Source: CAD feature listing. Evaluate the final solid. Frame: model axes, mm. A direction names the side the tool comes from. Coordinates: 2 decimals unless noted, no trailing zeros. Loops run counter-clockwise (first coordinate to the right, second up) from the corner with the lowest first, then second, coordinate; pieces in that order, holes last.
from build123d import *

# Parameters (mm, degrees)
SKETCH1_R               = 1.6
BOSS_EXTRUDE1_DEPTH     = 17
SKETCH2_R               = 1.65
CUT_EXTRUDE1_DEPTH      = 18
BOSS_EXTRUDE2_OUTLINE_R = 1.6
BOSS_EXTRUDE2_OUTLINE_W = 18.2
BOSS_EXTRUDE2_OUTLINE_H = 15.5
BOSS_EXTRUDE2_DEPTH     = 5
SKETCH5_R               = 8.1
CUT_EXTRUDE2_DEPTH      = 3
SKETCH6_R               = 4.5
CUT_EXTRUDE3_DEPTH      = 96.845918014
BOSS_EXTRUDE4_DEPTH     = 14
BOSS_EXTRUDE5_DEPTH     = 3
FILLET1_R               = 2
SKETCH10_W              = 9
SKETCH10_H              = 15
CUT_EXTRUDE4_DEPTH      = 5
FILLET2_R               = 1
FILLET3_R               = 1
FILLET4_R               = 2


# Read off the part's stored shape, not the designer's step: Boss-Extrude2
with BuildPart() as part:
    # Sketch1 → Boss-Extrude1 (new body)
    with BuildSketch(Plane.XY):
        with BuildLine():
            Line((10, -87.5), (10, -90))
            Line((10, -90), (26.2, -90))
            Line((26.2, -90), (26.2, 0))
            ThreePointArc((26.2, 0), (0, 26.2), (-26.2, 0))
            Line((-26.2, 0), (-26.2, -90))
            Line((-26.2, -90), (-10, -90))
            Line((-10, -90), (-10, -87.5))
            Line((-10, -87.5), (10, -87.5))
        make_face()
        with Locations((-23.7, -87.5)):
            Circle(SKETCH1_R, mode=Mode.SUBTRACT)
        with Locations((23.7, -87.5)):
            Circle(SKETCH1_R, mode=Mode.SUBTRACT)
        with Locations((-23.7, 0)):
            Circle(SKETCH1_R, mode=Mode.SUBTRACT)
        with Locations((0, 23.7)):
            Circle(SKETCH1_R, mode=Mode.SUBTRACT)
        with Locations((23.7, 0)):
            Circle(SKETCH1_R, mode=Mode.SUBTRACT)
        with BuildLine():
            Line((-21.2, -85), (21.2, -85))
            Line((21.2, -85), (21.2, 0))
            ThreePointArc((21.2, 0), (0, 21.2), (-21.2, 0))
            Line((-21.2, 0), (-21.2, -85))
        make_face(mode=Mode.SUBTRACT)
    extrude(amount=BOSS_EXTRUDE1_DEPTH)

    # Sketch2 → Cut-Extrude1 (cut)
    with BuildSketch(Plane.XZ.offset(90)):
        with Locations((15.5, 11.5)):
            Circle(SKETCH2_R)
        with Locations((-15.5, 11.5)):
            Circle(SKETCH2_R)
    extrude(amount=-CUT_EXTRUDE1_DEPTH, mode=Mode.SUBTRACT)

    # Boss-Extrude2 outline → Boss-Extrude2 (add)
    with BuildSketch(Plane.XY.offset(17)):
        with BuildLine():
            Line((-10, -87.5), (10, -87.5))
            Line((10, -87.5), (10, -90))
            Line((10, -90), (26.2, -90))
            Line((26.2, -90), (26.2, 0))
            ThreePointArc((26.2, 0), (0, 26.2), (-26.2, 0))
            Line((-26.2, 0), (-26.2, -90))
            Line((-26.2, -90), (-10, -90))
            Line((-10, -90), (-10, -87.5))
        make_face()
        with Locations((-23.7, -87.5)):
            Circle(BOSS_EXTRUDE2_OUTLINE_R, mode=Mode.SUBTRACT)
        with Locations((0, -77.25)):
            Rectangle(BOSS_EXTRUDE2_OUTLINE_W, BOSS_EXTRUDE2_OUTLINE_H, mode=Mode.SUBTRACT)
        with Locations((23.7, -87.5)):
            Circle(BOSS_EXTRUDE2_OUTLINE_R, mode=Mode.SUBTRACT)
        with Locations((-23.7, 0)):
            Circle(BOSS_EXTRUDE2_OUTLINE_R, mode=Mode.SUBTRACT)
        with Locations((0, 23.7)):
            Circle(BOSS_EXTRUDE2_OUTLINE_R, mode=Mode.SUBTRACT)
        with Locations((23.7, 0)):
            Circle(BOSS_EXTRUDE2_OUTLINE_R, mode=Mode.SUBTRACT)
    extrude(amount=BOSS_EXTRUDE2_DEPTH)

    # Sketch5 → Cut-Extrude2 (cut)
    with BuildSketch(Plane(origin=(0, 0, 17), x_dir=(-1, 0, 0), z_dir=(0, 0, -1))):
        with Locations((-12.995105527, -36.242762456)):
            Circle(SKETCH5_R)
    extrude(amount=-CUT_EXTRUDE2_DEPTH, mode=Mode.SUBTRACT)

    # Sketch6 → Cut-Extrude3 (cut, through all)
    with BuildSketch(Plane(origin=(0, 0, 20), x_dir=(-1, 0, 0), z_dir=(0, 0, -1))):
        with Locations((-12.995105527, -36.242762456)):
            Circle(SKETCH6_R)
    extrude(amount=-CUT_EXTRUDE3_DEPTH, mode=Mode.SUBTRACT)

    # Sketch7 → Boss-Extrude4 (add)
    with BuildSketch(Plane(origin=(0, 0, 17), x_dir=(-1, 0, 0), z_dir=(0, 0, -1))):
        with BuildLine():
            Line((21.2, -41), (13.2, -41))
            ThreePointArc((13.2, -41), (12.492893219, -40.707106781), (12.2, -40))
            Line((12.2, -40), (12.2, -20.899760764))
            ThreePointArc((12.2, -20.899760764), (10.968430418, -21.571590905), (9.7, -22.170926909))
            Line((9.7, -22.170926909), (9.7, -22.383029286))
            Line((9.7, -22.383029286), (9.7, -42.5))
            ThreePointArc((9.7, -42.5), (9.992893219, -43.207106781), (10.7, -43.5))
            Line((10.7, -43.5), (21.2, -43.5))
            Line((21.2, -43.5), (21.2, -41))
        make_face()
    extrude(amount=BOSS_EXTRUDE4_DEPTH)

    # Sketch8 → Boss-Extrude5 (add)
    with BuildSketch(Plane(origin=(0, 0, 3), x_dir=(-1, 0, 0), z_dir=(0, 0, -1))):
        with BuildLine():
            Line((12.2, -20.899760764), (21.2, -20.899760764))
            Line((21.2, -20.899760764), (21.2, -41))
            Line((21.2, -41), (21.2, -43.5))
            Line((21.2, -43.5), (10.7, -43.5))
            ThreePointArc((10.7, -43.5), (9.992893219, -43.207106781), (9.7, -42.5))
            Line((9.7, -42.5), (9.7, -22.170926909))
            ThreePointArc((9.7, -22.170926909), (10.968430418, -21.571590905), (12.2, -20.899760764))
        make_face()
    extrude(amount=BOSS_EXTRUDE5_DEPTH)

    # Fillet1
    # the kernel refuses this fillet: 2 mm, written as the material it takes off along each edge
    with BuildSketch(Plane(origin=(26.2, -95, 22), x_dir=(0, 0, -1), z_dir=(0, 1, 0)), Plane(origin=(-26.2, 0, 22), x_dir=(0, 0, -1), z_dir=(0, -1, 0))) as fillet1_piece_1:
        with BuildLine():
            CenterArc((FILLET1_R, FILLET1_R), FILLET1_R, 180, 90)
            Line((0, FILLET1_R), (0, 0))
            Line((0, 0), (FILLET1_R, 0))
        make_face()
    extrude(amount=95, mode=Mode.SUBTRACT)
    with BuildSketch(Plane(origin=(0, 0, 22), x_dir=(1, 0, 0), z_dir=(0, -1, 0))) as fillet1_piece_2:
        with BuildLine():
            CenterArc((26.2 - FILLET1_R, -FILLET1_R), FILLET1_R, 0, 90)
            Line((26.2, -FILLET1_R), (26.2, 0))
            Line((26.2, 0), (26.2 - FILLET1_R, 0))
        make_face()
    revolve(axis=Axis((0, 0, 22), (0, 0, 1)), revolution_arc=180, mode=Mode.SUBTRACT)

    # Sketch10 → Cut-Extrude4 (cut)
    with BuildSketch(Plane.XY.offset(22)):
        with Locations((-16.7, -33.5)):
            Rectangle(SKETCH10_W, SKETCH10_H)
    extrude(amount=-CUT_EXTRUDE4_DEPTH, mode=Mode.SUBTRACT)

    # Fillet2
    fillet2_edges = [part.edges().sort_by_distance(p)[0] for p in [
        (-21.2, -41, 12.5),
        (-12.2, -26, 19.5),
        (-21.2, -26, 19.5),
        (-12.2, -41, 19.5),
    ]]
    fillet(fillet2_edges, radius=FILLET2_R)

    # Fillet3
    fillet3_edges = [part.edges().sort_by_distance(p)[0] for p in [
        (-21.2, -43.5, 8.5),
        (-9.7, -32.335463454, 17),
        (-9.992893219, -43.207106781, 17),
        (-15.95, -43.5, 17),
        (-21.2, -20.899760764, 1.5),
    ]]
    fillet(fillet3_edges, radius=FILLET3_R)

    # Fillet4
    fillet4_edges = [part.edges().sort_by_distance(p)[0] for p in [
        (9.1, -69.5, 19.5),
        (-9.1, -69.5, 19.5),
    ]]
    fillet(fillet4_edges, radius=FILLET4_R)


solid = part.part
Q1. Line query: line 1 along Y through (x, z) = (0, 9); line 2 along X through (y, z) = (-18, 6); line 3 along Z through (x, y) = (15.5, -87.5). Output: solid intervals per line, ascending.
Q2. Access query for faces 5 (the flat face through (-17, -41, 13)), 6 (the flat face through (10, -89, 11)), 7 (the cylindrical face through (-8.5, -70.07, 19.54)), 8 (the cylindrical face through (0.466, 21.195, 8.381)). Directions: +Z, -Z, +X, -X, +Y, -Y. A direction counts if a zero-diameter tool reaches every point of the face in a straight line with its end or side. Return the directions, or none.
Q3. Section A-A, the plane z = 6.75. Return the cut outline in (x, y), plus the area to 3 significant figures.
Q4. Section C-C, the plane z = 11.5. Count the separate pieces of the cut face and the enclosed holes in it, plus the area to 3 significant figures.
Q5. Contact query for flat-ended pins moving along their axis: pin 1 Ø11.5 at (x, y) = (13, -36.24) entering from -Z; pin 2 Ø0.9 at (x, z) = (-16, 2) entering from +Y; pin 3 Ø21 at (x, y) = (3, -28) entering from -Z. Output: stop coordinate, or through.
Q6. Section B-B, the plane x = 0. Return the cut outline in (y, z).
Q7. Draft query along X for faces 1 (the cylindrical face through (25.226, 0.481, 10.846)), 2 (the flat face through (26.2, -46, 10)), 3 (the cylindrical face through (-25.3, 0.07, 10.85)), 4 (the flat face through (-18, -90, 11)). Return one class per face: +X half, -X half, draft (parallel to the pull), parting line (faces both ways), or undercut.
Derived:
1. line 1: y = -87.5 to -85, 21.2 to 22.1, 25.3 to 26.2
1. line 2: x = -26.2 to -21.2, 21.2 to 26.2
1. line 3: z = 0 to 9.85, 13.15 to 22
2. face 5: +Z
2. face 6: +Z, -Z, -Y
2. face 7: +Z, -Z
2. face 8: -Z
3. outline: (-26.2, -90) - (-10, -90) - (-10, -87.5) - (10, -87.5) - (10, -90) - (26.2, -90) - (26.2, 0) arc R26.2 ccw to (-26.2, 0) - close; hole circle Ø3.2 at (-23.7, -87.5); hole circle Ø3.2 at (-23.7, 0); hole (-21.2, -85) - (21.2, -85) - (21.2, 0) arc R21.2 ccw to (-21.2, 0) - (-21.2, -40) arc R1 ccw to (-20.2, -41) - (-13.2, -41) arc R1 ccw to (-12.2, -40) - (-12.2, -20.9) arc R24.2 ccw to (-9.7, -22.17) - (-9.7, -42.5) arc R1 cw to (-10.7, -43.5) - (-20.2, -43.5) arc R1 ccw to (-21.2, -44.5) - close; hole circle Ø3.2 at (0, 23.7); hole circle Ø3.2 at (23.7, -87.5); hole circle Ø3.2 at (23.7, 0)
3. area: 1,470 mm2
4. separate pieces: 2
4. enclosed holes: 5
4. area: 1,440 mm2
5. pin 1: stops at z = 20
5. pin 2: stops at y = 21.09
5. pin 3: stops at z = 17
6. outline: (-87.5, 0) - (-85, 0) - (-85, 22) - (-87.5, 22) - close; (-69.5, 17) - (21.2, 17) - (21.2, 0) - (22.1, 0) - (22.1, 22) - (-69.5, 22) - close; (25.3, 0) - (26.2, 0) - (26.2, 20) arc R2 ccw to (25.3, 21.67) - close
7. face 1: undercut
7. face 2: +X half
7. face 3: undercut
7. face 4: draft
